from build123d import *

# Parameters (mm, degrees)
F0_R           = 225
F0_R_2         = 200
F1_DEPTH       = 17
F3_D           = 5.5
F3_CBORE_D     = 10
F3_CBORE_DEPTH = 5.4
F4_R           = 3
F6_DEPTH       = 17.001


# Not quite as in the source:
# - a feature names something its author has since deleted; it is built from what else it names


with BuildPart() as f1:
    # F0 (on Top) → F1 (new body)
    with BuildSketch(Plane.XY):
        Circle(F0_R)
        Circle(F0_R_2, mode=Mode.SUBTRACT)
    extrude(amount=F1_DEPTH)

    # F3 (through all)
    with Locations(Plane.XY.offset(17)):
        with Locations((219, 0), (205.7926839521, 74.9024113883), (167.7637330431, 140.7704865214), (109.5, 189.6595634288), (38.0289509091, 215.6728979097), (-38.0289509091, 215.6728979097), (-109.5, 189.6595634288), (-167.7637330431, 140.7704865214), (-205.7926839521, 74.9024113883), (-219, 0), (-205.7926839521, -74.9024113883), (-167.7637330431, -140.7704865214), (-109.5, -189.6595634288), (-38.0289509091, -215.6728979097), (38.0289509091, -215.6728979097), (109.5, -189.6595634288), (167.7637330431, -140.7704865214), (205.7926839521, -74.9024113883)):
            CounterBoreHole(F3_D / 2, F3_CBORE_D / 2, F3_CBORE_DEPTH)

    # F4
    f4_edges = [f1.edges().sort_by_distance(p)[0] for p in [
        (-200, 0, 0),
    ]]
    fillet(f4_edges, radius=F4_R)

    # F5 (on face) → F6 (cut, through all)
    with BuildSketch(Plane.XY.offset(17)):
        with BuildLine():
            ThreePointArc((223.6935148816, 24.2118029049), (221.5817444277, 39.0708399751), (218.4840695516, 53.7560354952))
            Line((218.4840695516, 53.7560354952), (208.6359920215, 52.0195537186))
            ThreePointArc((208.6359920215, 52.0195537186), (207.3449842883, 51.1970910852), (207.0136728708, 49.7026418572))
            Line((207.0136728708, 49.7026418572), (209.2710991805, 36.900141068))
            Line((209.2710991805, 36.900141068), (211.5285254901, 24.0976402789))
            ThreePointArc((211.5285254901, 24.0976402789), (212.3509881235, 22.8066325456), (213.8454373515, 22.4753211282))
            Line((213.8454373515, 22.4753211282), (223.6935148816, 24.2118029049))
        make_face()
        with BuildLine():
            Line((149.3682510245, 154.6742923751), (155.7961271214, 162.3347368063))
            ThreePointArc((155.7961271214, 162.3347368063), (144.6272121795, 172.3599997018), (132.8147938278, 181.6183650969))
            Line((132.8147938278, 181.6183650969), (126.386917731, 173.9579206657))
            ThreePointArc((126.386917731, 173.9579206657), (125.926617221, 172.4980339608), (126.6334313978, 171.1402565601))
            Line((126.6334313978, 171.1402565601), (136.5920091584, 162.7840176342))
            Line((136.5920091584, 162.7840176342), (146.5505869189, 154.4277787082))
            ThreePointArc((146.5505869189, 154.4277787082), (148.0104736238, 153.9674781983), (149.3682510245, 154.6742923751))
        make_face()
        with BuildLine():
            Line((15, 214.4994432064), (15, 224.4994432064))
            ThreePointArc((15, 224.4994432064), (0, 225), (-15, 224.4994432064))
            Line((-15, 224.4994432064), (-15, 214.4994432064))
            ThreePointArc((-15, 214.4994432064), (-14.4142135624, 213.0852296441), (-13, 212.4994432064))
            Line((-13, 212.4994432064), (0, 212.4994432064))
            Line((0, 212.4994432064), (13, 212.4994432064))
            ThreePointArc((13, 212.4994432064), (14.4142135624, 213.0852296441), (15, 214.4994432064))
        make_face()
        with BuildLine():
            Line((-126.386917731, 173.9579206657), (-132.8147938278, 181.6183650969))
            ThreePointArc((-132.8147938278, 181.6183650969), (-144.6272121795, 172.3599997018), (-155.7961271214, 162.3347368063))
            Line((-155.7961271214, 162.3347368063), (-149.3682510245, 154.6742923751))
            ThreePointArc((-149.3682510245, 154.6742923751), (-148.0104736238, 153.9674781983), (-146.5505869189, 154.4277787082))
            Line((-146.5505869189, 154.4277787082), (-136.5920091584, 162.7840176342))
            Line((-136.5920091584, 162.7840176342), (-126.6334313978, 171.1402565601))
            ThreePointArc((-126.6334313978, 171.1402565601), (-125.926617221, 172.4980339608), (-126.386917731, 173.9579206657))
        make_face()
        with BuildLine():
            Line((-208.6359920215, 52.0195537186), (-218.4840695516, 53.7560354952))
            ThreePointArc((-218.4840695516, 53.7560354952), (-221.5817444277, 39.0708399751), (-223.6935148816, 24.2118029049))
            Line((-223.6935148816, 24.2118029049), (-213.8454373515, 22.4753211282))
            ThreePointArc((-213.8454373515, 22.4753211282), (-212.3509881235, 22.8066325456), (-211.5285254901, 24.0976402789))
            Line((-211.5285254901, 24.0976402789), (-209.2710991805, 36.900141068))
            Line((-209.2710991805, 36.900141068), (-207.0136728708, 49.7026418572))
            ThreePointArc((-207.0136728708, 49.7026418572), (-207.3449842883, 51.1970910852), (-208.6359920215, 52.0195537186))
        make_face()
        with BuildLine():
            ThreePointArc((-201.9222209522, -99.2593405465), (-194.8557158515, -112.5), (-186.9222209522, -125.24010266))
            Line((-186.9222209522, -125.24010266), (-178.2619669144, -120.24010266))
            ThreePointArc((-178.2619669144, -120.24010266), (-177.3301152618, -119.0256899426), (-177.5299161068, -117.5080518524))
            Line((-177.5299161068, -117.5080518524), (-184.0299161068, -106.2497216032))
            Line((-184.0299161068, -106.2497216032), (-190.5299161068, -94.991391354))
            ThreePointArc((-190.5299161068, -94.991391354), (-191.7443288242, -94.0595397014), (-193.2619669144, -94.2593405465))
            Line((-193.2619669144, -94.2593405465), (-201.9222209522, -99.2593405465))
        make_face()
        with BuildLine():
            ThreePointArc((-90.8787210538, -205.8301680017), (-76.9545322483, -211.4308396768), (-62.6879424302, -216.0907723015))
            Line((-62.6879424302, -216.0907723015), (-59.267740997, -206.6938460937))
            ThreePointArc((-59.267740997, -206.6938460937), (-59.3345106645, -205.1645692835), (-60.4630859519, -204.1304205654))
            Line((-60.4630859519, -204.1304205654), (-72.6790900221, -199.6841587022))
            Line((-72.6790900221, -199.6841587022), (-84.8950940923, -195.237896839))
            ThreePointArc((-84.8950940923, -195.237896839), (-86.4243709024, -195.3046665065), (-87.4585196205, -196.4332417939))
            Line((-87.4585196205, -196.4332417939), (-90.8787210538, -205.8301680017))
        make_face()
        with BuildLine():
            ThreePointArc((62.6879424302, -216.0907723015), (76.9545322483, -211.4308396768), (90.8787210538, -205.8301680017))
            Line((90.8787210538, -205.8301680017), (87.4585196205, -196.4332417939))
            ThreePointArc((87.4585196205, -196.4332417939), (86.4243709024, -195.3046665065), (84.8950940923, -195.237896839))
            Line((84.8950940923, -195.237896839), (72.6790900221, -199.6841587022))
            Line((72.6790900221, -199.6841587022), (60.4630859519, -204.1304205654))
            ThreePointArc((60.4630859519, -204.1304205654), (59.3345106645, -205.1645692835), (59.267740997, -206.6938460937))
            Line((59.267740997, -206.6938460937), (62.6879424302, -216.0907723015))
        make_face()
        with BuildLine():
            ThreePointArc((186.9222209522, -125.24010266), (194.8557158515, -112.5), (201.9222209522, -99.2593405465))
            Line((201.9222209522, -99.2593405465), (193.2619669144, -94.2593405465))
            ThreePointArc((193.2619669144, -94.2593405465), (191.7443288242, -94.0595397014), (190.5299161068, -94.991391354))
            Line((190.5299161068, -94.991391354), (184.0299161068, -106.2497216032))
            Line((184.0299161068, -106.2497216032), (177.5299161068, -117.5080518524))
            ThreePointArc((177.5299161068, -117.5080518524), (177.3301152618, -119.0256899426), (178.2619669144, -120.24010266))
            Line((178.2619669144, -120.24010266), (186.9222209522, -125.24010266))
        make_face()
    extrude(amount=-F6_DEPTH, mode=Mode.SUBTRACT)


solid = f1.part
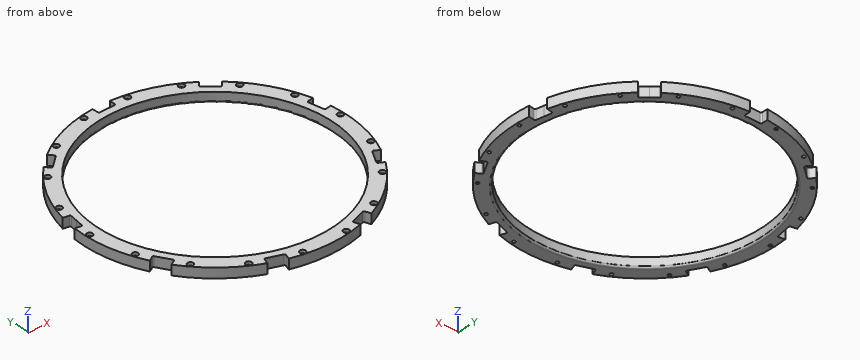
Read the model definition and answer for the solid it produces. Units are mm, in the model's axes. Give positions to 0.01 mm unless a question says otherwise; leave off trailing zeros. Loops run counter-clockwise (first coordinate to the right, second up) from the corner with the lowest first, then second, coordinate; pieces in that order, holes last. Notation, with made-up numbers: M 2,84.5 L 46,84.5 A11 cw 46,102.5 Z; hole C 59,80 d8. An arc over 180 degrees is marked long. Write each question's results on one line, items separated by ' | '.
1. Section A-A on x = 0 is taken. Give the vertices of the cut face in (y, z).
Values:
outline: M -225,0 L -203,0 A3 ccw -200,3 L -200,17 L -225,17 Z; M 200,3 A3 ccw 203,0 L 212.5,0 L 212.5,17 L 200,17 Z
2. Section B-B on z = 8.5 is taken. State how many separate pieces and enclosed holes the cut face has, plus the area to 3 significant figures.
Values:
separate pieces: 1 | enclosed holes: 19 | area: 29,600 mm^2
3. Straight lines are drawn through the part: line 1 (X direction, y = 4, z = 4.75); line 2 (Y direction, x = 109.5, z = 15.3); line 3 (X direction, y = 158, z = 2). For each, find the intervals that lie inside material, in ascending order. Write a range as [from, to].
Values:
line 1: x = [-224.96, -199.96], [199.96, 224.96] | line 2: y = [-196.56, -194.66], [-184.66, -167.36], [167.36, 184.66], [194.66, 196.56] | line 3: x = [-160.19, -152.16], [-142.29, -122.9], [122.9, 142.29], [152.16, 160.19]
4. Given pin 1 (1.5 mm diameter, centred on y = 70.5, z = 2.5, fed in from -X); pin 2 (3 mm diameter, centred on x = -10.5, z = 2.5, fed in from +Y); pin 3 (4.5 mm diameter, centred on x = 38.03, y = -215.67, fed in from +Z); pin 4 (1 mm diameter, centred on y = 102.5, z = 14.5, fed in from +X), each flat-ended and moving along its own axis, determine where each tip first touches the part or whether it passes through.
Values:
pin 1: stops at x = -213.92 | pin 2: stops at y = 212.5 | pin 3: passes through | pin 4: stops at x = 200.55
